Could you check a few things on this drawing? It's one solid part, dimensions in mm from its lowest x, y, z. A direction names the side the tool comes from. Give positions to 0.01 mm unless a question says otherwise; leave off trailing zeros. Loops run counter-clockwise (first coordinate to the right, second up) from the corner with the lowest first, then second, coordinate; pieces in that order, holes last.
1. Thinking about a two-plate mould opening in Z: for the marked faces 1, 2 and 3, which applies, +Z half, -Z half, draft (parallel to the pull), parting line (faces both ways), or undercut?
2. Imagine slicing it at B-B (z = 16.5). List the corners of the cut face in (x, y) for me.
3. Imagine slicing it at D-D (z = 45). List the corners of the cut face in (x, y) for me.
4. Imagine slicing it at C-C (x = 22.5). List the corners of the cut face in (y, z) for me.
5. Imagine slicing it at A-A (y = 27). List the corners of the cut face in (x, z) for me, plus the area to 3 significant figures.
6. I need wall thicknesses on line 1 along X through (y, z) = (52, 56); line 2 along X through (y, z) = (56.5, 23); line 3 along Y through (x, z) = (3.5, 53). Which ranges of each line are inside material? Lowest first, please.
7. For the marked faces 4, 5, 6, 7 and 8, which set-ups out of +Z, -Z, +X, -X, +Y, -Y let a thin tool reach every point of the face, with its end or its side?
8. For P1, Ø10, axis at x = 13.5, z = 44, coming from the +Y side; P2, Ø13, axis at x = 9, z = 41, coming from the +Y side; P3, Ø3, axis at y = 52.5, z = 76.5, coming from the +X side, each with a flat end and sliding along its axis, tell me the tip position at first contact or that it passes through.
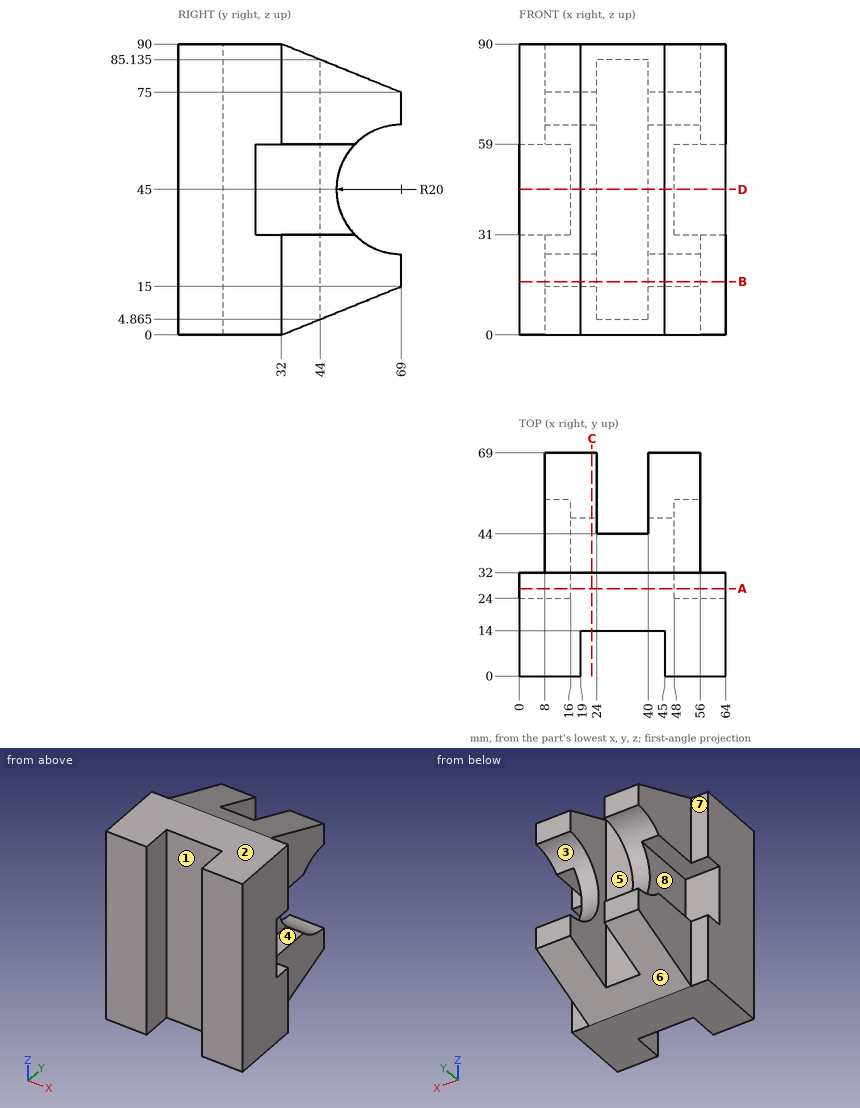
Derived:
1. face 1: draft
1. face 2: +Z half
1. face 3: undercut
2. outline: (0, 0) - (19, 0) - (19, 14) - (45, 14) - (45, 0) - (64, 0) - (64, 32) - (56, 32) - (56, 69) - (40, 69) - (40, 44) - (24, 44) - (24, 69) - (8, 69) - (8, 32) - (0, 32) - close
3. outline: (0, 0) - (19, 0) - (19, 14) - (45, 14) - (45, 0) - (64, 0) - (64, 24) - (48, 24) - (48, 49) - (40, 49) - (40, 44) - (24, 44) - (24, 49) - (16, 49) - (16, 24) - (0, 24) - close
4. outline: (14, 0) - (32, 0) - (69, 15) - (69, 25) arc R20 cw to (69, 65) - (69, 75) - (32, 90) - (14, 90) - close
5. outline: (0, 0) - (64, 0) - (64, 31) - (48, 31) - (48, 59) - (64, 59) - (64, 90) - (0, 90) - (0, 59) - (16, 59) - (16, 31) - (0, 31) - close
5. area: 4,860 mm2
6. line 1: x = 16 to 24, 40 to 48
6. line 2: x = 8 to 24, 40 to 56
6. line 3: y = 0 to 24
7. face 4: +X, +Y
7. face 5: +Z, -Z, +Y
7. face 6: -Z, +X, -X, +Y
7. face 7: +Z, -Z, -X, +Y
7. face 8: -X, +Y
8. P1: stops at y = 49.72
8. P2: stops at y = 24
8. P3: stops at x = 56
